```python
from build123d import *

# Parameters (mm, degrees)
BOSS_EXTRUDE1_DEPTH  = 5
SKETCH1_3_W          = 43.4
SKETCH1_3_H          = 57
CUT_EXTRUDE1_DEPTH   = 4
SKETCH4_W            = 43.4
SKETCH4_H            = 1
CUT_EXTRUDE2_DEPTH   = 0.8
SKETCH5_W            = 43.4
SKETCH5_H            = 1
CUT_EXTRUDE3_DEPTH   = 0.8
SKETCH6_W            = 58.6
SKETCH6_H            = 1
CUT_EXTRUDE4_DEPTH   = 0.8
FILLET1_R            = 1
SKETCH8_W            = 1.5
SKETCH8_H            = 1
BOSS_EXTRUDE2_DEPTH  = 0.5
FILLET2_R            = 0.5
FILLET2_OF_MIRROR1_R = 0.5


# Read off the part's stored shape, not the designer's step: Boss-Extrude1
with BuildPart() as part:
    # Boss-Extrude1 outline → Boss-Extrude1 (new body)
    with BuildSketch(Plane(origin=(0, 8.5, 0), x_dir=(1, 0, 0), z_dir=(0, 1, 0))):
        with BuildLine():
            Line((-23.5, -30), (20.4, -30))
            Line((20.4, -30), (20.4, 30))
            Line((20.4, 30), (-23.5, 30))
            ThreePointArc((-23.5, 30), (-24.207106781, 29.707106781), (-24.5, 29))
            Line((-24.5, 29), (-24.5, -29))
            ThreePointArc((-24.5, -29), (-24.207106781, -29.707106781), (-23.5, -30))
        make_face()
    extrude(amount=BOSS_EXTRUDE1_DEPTH)

    # Sketch1<3> → Cut-Extrude1 (cut)
    with BuildSketch(Plane(origin=(0, 8.5, 0), x_dir=(1, 0, 0), z_dir=(0, 1, 0))):
        with Locations((-1.3, 0)):
            Rectangle(SKETCH1_3_W, SKETCH1_3_H)
    extrude(amount=CUT_EXTRUDE1_DEPTH, mode=Mode.SUBTRACT)

    # Sketch4 → Cut-Extrude2 (cut)
    with BuildSketch(Plane.XY.offset(-28.5)):
        with Locations((-1.3, 11)):
            Rectangle(SKETCH4_W, SKETCH4_H)
    extrude(amount=-CUT_EXTRUDE2_DEPTH, mode=Mode.SUBTRACT)

    # Sketch5 → Cut-Extrude3 (cut)
    with BuildSketch(Plane(origin=(0, 0, 28.5), x_dir=(-1, 0, 0), z_dir=(0, 0, -1))):
        with Locations((1.3, 11)):
            Rectangle(SKETCH5_W, SKETCH5_H)
    extrude(amount=-CUT_EXTRUDE3_DEPTH, mode=Mode.SUBTRACT)

    # Sketch6 → Cut-Extrude4 (cut)
    with BuildSketch(Plane(origin=(-23, 0, 0), x_dir=(0, 0, -1), z_dir=(1, 0, 0))):
        with Locations((0, 11)):
            Rectangle(SKETCH6_W, SKETCH6_H)
    extrude(amount=-CUT_EXTRUDE4_DEPTH, mode=Mode.SUBTRACT)

    # Fillet1
    fillet1_edges = [part.edges().sort_by_distance(p)[0] for p in [
        (-1.55, 13.5, -30),
        (-24.207106781, 13.5, -29.707106781),
        (-24.5, 13.5, 0),
        (-24.207106781, 13.5, 29.707106781),
        (-1.55, 13.5, 30),
    ]]
    fillet(fillet1_edges, radius=FILLET1_R)

    # Sketch8 → Boss-Extrude2 (add)
    with BuildSketch(Plane(origin=(0, 0, 29.3), x_dir=(-1, 0, 0), z_dir=(0, 0, -1))):
        with Locations((-17.785673559, 11)):
            Rectangle(SKETCH8_W, SKETCH8_H)
    boss_extrude2 = extrude(amount=BOSS_EXTRUDE2_DEPTH)

    # Fillet2
    fillet2_edges = [part.edges().sort_by_distance(p)[0] for p in [
        (18.535673559, 11, 28.8),
        (17.035673559, 11, 28.8),
    ]]
    fillet(fillet2_edges, radius=FILLET2_R - 0.0001)  # a hair under: the kernel refuses the full size

    # Mirror1: Boss-Extrude2 across plane
    add(boss_extrude2.mirror(Plane(origin=(0, 0, 0), x_dir=(1, 0, 0), z_dir=(0, 0, -1))))

    # Fillet2 of Mirror1
    fillet2_of_mirror1_edges = [part.edges().sort_by_distance(p)[0] for p in [
        (18.535673559, 11, -28.8),
        (17.035673559, 11, -28.8),
    ]]
    fillet(fillet2_of_mirror1_edges, radius=FILLET2_OF_MIRROR1_R - 0.0001)  # a hair under: the kernel refuses the full size


solid = part.part
```
Can you work these out from the model? Positions are in its coordinate system, mm. A direction names the side the tool comes from. Coordinates: 2 decimals unless noted, no trailing zeros. Write each loop counter-clockwise with the first axis right and the second up, starting at its lowest first coordinate (ties: lowest second). Pieces come first, ordered by that corner, then holes. Notation, with made-up numbers: M -31,11.25 L -16,11.25 A21 ccw -16,44.25 Z; hole C 66,37.5 d7. An arc over 180 degrees is marked long. Write item = value, one per line. Start each with the question number.
Q1. Thinking about a two-plate mould opening in Z: for faces 3 (the face through (-2, 10, 30)), 4 (the face through (-1, 10, -30)), 5 (the face through (-24.5, 10, 0)), 6 (the face through (-2, 12.5, 0)), which applies, released by +Z, released by -Z, zero draft, split by the parting line, or undercut?
Q2. If we section it at B-B, the plane x = 4.5: Write out the boundary of the cut face in (y, z).
Q3. I'm going to push flat-ended pins straight in: pin 1 (1 mm diameter, centred on x = -11.5, z = 10, fed in from -Y); pin 2 (0.8 mm diameter, centred on y = 11, z = -10, fed in from +X); pin 3 (1.6 mm diameter, centred on y = 9.5, z = -2, fed in from +X). Where does each tip first touch, or does it pass through?
Q4. If we section it at A-A, the plane z = -12: Write out the boundary of the cut face in (x, y).
Q5. If I drill on L1, parallel to Z at x = -3, y = 11; L2, parallel to Z at x = 15, y = 9.8; L3, parallel to X at y = 8.8, z = -7.5, over which ranges is the centre line in solid material (lowest first)? Write a range as [from, to].
Q6. On a 3-axis mill with a long thin cutter (end or side, diameter ignored), from which of +Z, -Z, +X, -X, +Y, -Y can I reach the whole of each face in a straight line? I mean faces 1 (the face through (-23, 9, 0)), 2 (the face through (-2, 13.5, 0)). Say none if no direction works.
Check sheet entries:
q1.face_3 = released by +Z
q1.face_4 = released by -Z
q1.face_5 = zero draft
q1.face_6 = undercut
q2.outline = M 8.5,-30 L 12.5,-30 A1 ccw 13.5,-29 L 13.5,29 A1 ccw 12.5,30 L 8.5,30 L 8.5,28.5 L 10.5,28.5 L 10.5,29.3 L 11.5,29.3 L 11.5,28.5 L 12.5,28.5 L 12.5,-28.5 L 11.5,-28.5 L 11.5,-29.3 L 10.5,-29.3 L 10.5,-28.5 L 8.5,-28.5 Z
q3.pin_1 = 12.5
q3.pin_2 = -23.8
q3.pin_3 = -23
q4.outline = M -24.5,8.5 L -23,8.5 L -23,10.5 L -23.8,10.5 L -23.8,11.5 L -23,11.5 L -23,12.5 L 20.4,12.5 L 20.4,13.5 L -23.5,13.5 A1 ccw -24.5,12.5 Z
q5.L1 = [-30, -29.3], [29.3, 30]
q5.L2 = [-30, -28.5], [28.5, 30]
q5.L3 = [-24.5, -23]
q6.face_1 = +X, -Y
q6.face_2 = +Z, -Z, +X, -X, +Y
